Build history of the part. All positions in model axes, mm. A direction names the side the tool comes from. Round coordinates to 2 decimals unless told otherwise and drop trailing zeros. Order: outer loops, then holes, each group sorted by start corner. A loop starts at its lowest first (then second) coordinate and runs counter-clockwise, first axis right, second up. Notation, with made-up numbers: (25.25, -4) -> (45.25, -4) arc R34 ccw to (45.25, 34) -> close; hole circle Ø9 at (16.25, -32.5). An arc over 180 degrees is marked (long way). Use a Markdown table: item, result. Add a question column.
Item 1: Two-plate mould, pull along Z, no slides. Class faces 1 (the face through (-81.359, 1.479, 26.797)), 2 (the face through (45, 1, 0)), 3 (the face through (82.5, 1, 0)): released by +Z, released by -Z, zero draft, split by the parting line, or undercut.
Item 2: Probe L1, parallel to X at y = 1.1, z = -3; L2, parallel to X at y = 0.85, z = -24.5. List the from-to ranges inside material, lowest first.
Item 3: 3-axis set-ups, long thin cutter, end or side, ignore diameter. For faces 4 (the face through (-44, 1, -11)), 5 (the face through (-1, 1, 28)): which of +Z, -Z, +X, -X, +Y, -Y reach the whole face in a straight line?
Item 4: Slice it at B-B, the plane z = -2.5. Give the cut face in (x, y).
Item 5: Slice it at A-A, the plane y = 1.1. Give the cut face in (x, z), plus the area to 3 significant figures.
from build123d import *

# Parameters (mm, degrees)
BOSS_EXTRUDE1_DEPTH     = 3
CUT_EXTRUDE1_DEPTH      = 88.17367722
CUT_EXTRUDE1_DEPTH_BACK = 88.17367722
SKETCH2_W               = 3
SKETCH2_H               = 22


with BuildPart() as part:
    # Sketch1 → Boss-Extrude1 (new body)
    with BuildSketch(Plane(origin=(0, 0, 0), x_dir=(1, 0, 0), z_dir=(0, 1, 0))):
        with BuildLine():
            Line((-78.5, -28), (78.5, -28))
            ThreePointArc((78.5, -28), (81.328427125, -26.828427125), (82.5, -24))
            Line((82.5, -24), (82.5, 24))
            ThreePointArc((82.5, 24), (81.328427125, 26.828427125), (78.5, 28))
            Line((78.5, 28), (-78.5, 28))
            ThreePointArc((-78.5, 28), (-81.328427125, 26.828427125), (-82.5, 24))
            Line((-82.5, 24), (-82.5, -24))
            ThreePointArc((-82.5, -24), (-81.328427125, -26.828427125), (-78.5, -28))
        make_face()
    extrude(amount=BOSS_EXTRUDE1_DEPTH)

    # Sketch2 → Cut-Extrude1 (cut, two sides: drawn at the far end of the back side and taken through both)
    with BuildSketch(Plane(origin=(0, 0, 0), x_dir=(1, 0, 0), z_dir=(0, 1, 0)).offset(-CUT_EXTRUDE1_DEPTH_BACK)):
        with Locations((-43.5, 0)):
            Rectangle(SKETCH2_W, SKETCH2_H)
        with Locations((43.5, 0)):
            Rectangle(SKETCH2_W, SKETCH2_H)
    extrude(amount=CUT_EXTRUDE1_DEPTH + CUT_EXTRUDE1_DEPTH_BACK, mode=Mode.SUBTRACT)


solid = part.part
Check sheet entries:
| question | item | result |
|---|---|---|
| 1 | face 1 | released by +Z |
| 1 | face 2 | undercut |
| 1 | face 3 | zero draft |
| 2 | L1 | -82.5 to -45, -42 to 42, 45 to 82.5 |
| 2 | L2 | -82.47 to 82.47 |
| 3 | face 4 | +Y, -Y |
| 3 | face 5 | +Z, +X, -X, +Y, -Y |
| 4 | outline | (-82.5, 0) -> (-45, 0) -> (-45, 3) -> (-82.5, 3) -> close; (-42, 0) -> (42, 0) -> (42, 3) -> (-42, 3) -> close; (45, 0) -> (82.5, 0) -> (82.5, 3) -> (45, 3) -> close |
| 5 | outline | (-82.5, -24) arc R4 ccw to (-78.5, -28) -> (78.5, -28) arc R4 ccw to (82.5, -24) -> (82.5, 24) arc R4 ccw to (78.5, 28) -> (-78.5, 28) arc R4 ccw to (-82.5, 24) -> close; hole (-45, -11) -> (-42, -11) -> (-42, 11) -> (-45, 11) -> close; hole (42, -11) -> (45, -11) -> (45, 11) -> (42, 11) -> close |
| 5 | area | 9,090 mm2 |
